Geometry check sheet. Reference: the model listing, model coordinates, mm. Face numbers are marked on the shaded views. A direction names the side the tool comes from. Coordinates: 2 decimals unless noted, no trailing zeros. Loops run counter-clockwise (first coordinate to the right, second up) from the corner with the lowest first, then second, coordinate; pieces in that order, holes last. Notation, with made-up numbers: (-23.75, 29) -> (10.25, 29) arc R19 ccw to (10.25, 34) -> close; hole circle Ø2 at (32, -6.5). An arc over 180 degrees is marked (long way). Answer as a JSON object with one key per item and string values.
Autodesk Inventor part; units mm, degrees
ref_plane "YZ Plane" through (0, 0, 0) normal (1, 0, 0) x (0, 1, 0)
ref_plane "XZ Plane" through (0, 0, 0) normal (0, 1, 0) x (-1, 0, 0)
ref_plane "XY Plane" through (0, 0, 0) normal (0, 0, 1) x (1, 0, 0)
sketch "Sketch1" plane through (0, 0, 0) normal (0, 0, 1) x (1, 0, 0)
  line L0 (0, 0) -> (0, 21)
  arc A0 (3.873, 18) -> (0, 21) centre (0, 17) ccw
  line L1 (3.873, 18) -> (2, 18)
  line L2 (2, 18) -> (2, 0)
  line L3 (2, 0) -> (0, 0)
  dimension "Diameter" = 4
  dimension "Length" = 18
  dimension "d2" = 4
  dimension "d3" = 3
revolve "Revolution1" add sketch "Sketch1" angle 360 about axis through (0, 0, 0) along (0, 1, 0)
thread "Thread1"
sketch "Sketch2" plane through (0, 0, 0) normal (1, 0, 0) x (0, 1, 0)
  arc A0 (18, -3.873) -> (18, 3.873) centre (17, 0) ccw construction
  line L0 (0, 0) -> (21, 0) construction
  line L1 (21, 0.5) -> (19, 0.5)
  line L2 (19, 0.5) -> (19, -0.5)
  line L3 (19, -0.5) -> (21, -0.5)
  line L4 (21, -0.5) -> (21, 0.5)
  dimension "d7" = 2
  dimension "d8" = 1
extrude "Extrusion1" cut sketch "Sketch2" along normal through all both and the other way through all
chamfer "Chamfer1" distance 0.5 angle 45 1 edges at (-2, 0, 0)
equation "\"d2\" = Diameter"
equation "\"d3\" = 0.75 * Diameter"
equation "\"d7\" = 0.5 * Diameter"
equation "\"d8\" = 0.25 * Diameter"
properties part number "Round Head Machine Screw"
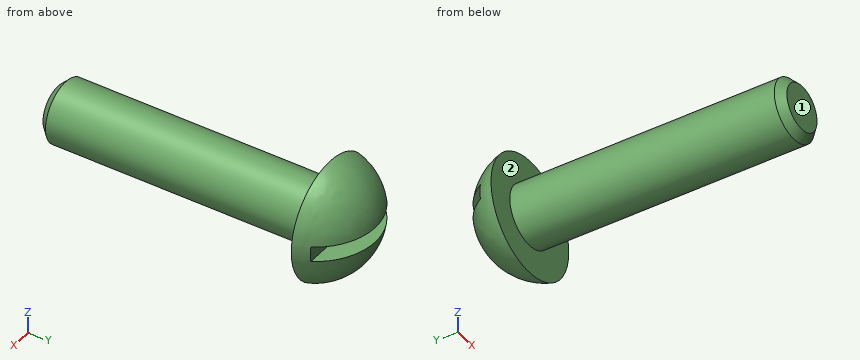
1. Section check A-A, the plane y = 9.75. Record the boundary of the cut face in (x, z), then the cut area to 3 significant figures.
Evaluation:
{"outline": "circle Ø4 at (0, 0)", "area": "12.6 mm^2"}
2. Depth check by flat-ended pin: P1, Ø2, axis at x = 0, y = 20.5, coming from the -Z side; P2, Ø4, axis at y = 11.5, z = -0.5, coming from the -X side; P3, Ø0.5, axis at x = 1.5, z = 0, coming from the +Y side. Enter the tip coordinate at first touch or a pass-through.
Evaluation:
{"P1": "stops at z = -3.12", "P2": "stops at x = -2", "P3": "stops at y = 19"}
3. Thickness scan on probe 1 along Y at (x, z) = (-0.25, 0); probe 2 along Y at (x, z) = (2.75, 0); probe 3 along Z at (x, y) = (1.25, 12.25). Record the ranges inside material, lowest first. Write a range as from..to.
Evaluation:
{"probe 1": "y = 0..19", "probe 2": "y = 18..19", "probe 3": "z = -1.56..1.56"}
4. Tool access check on the marked faces 1 and 2. Record the directions out of +Z, -Z, +X, -X, +Y, -Y that give a thin tool (end or side, any length) a straight path to the whole face; none if there is none.
Evaluation:
{"face 1": "+Z, -Z, +X, -X, -Y", "face 2": "-Y"}
